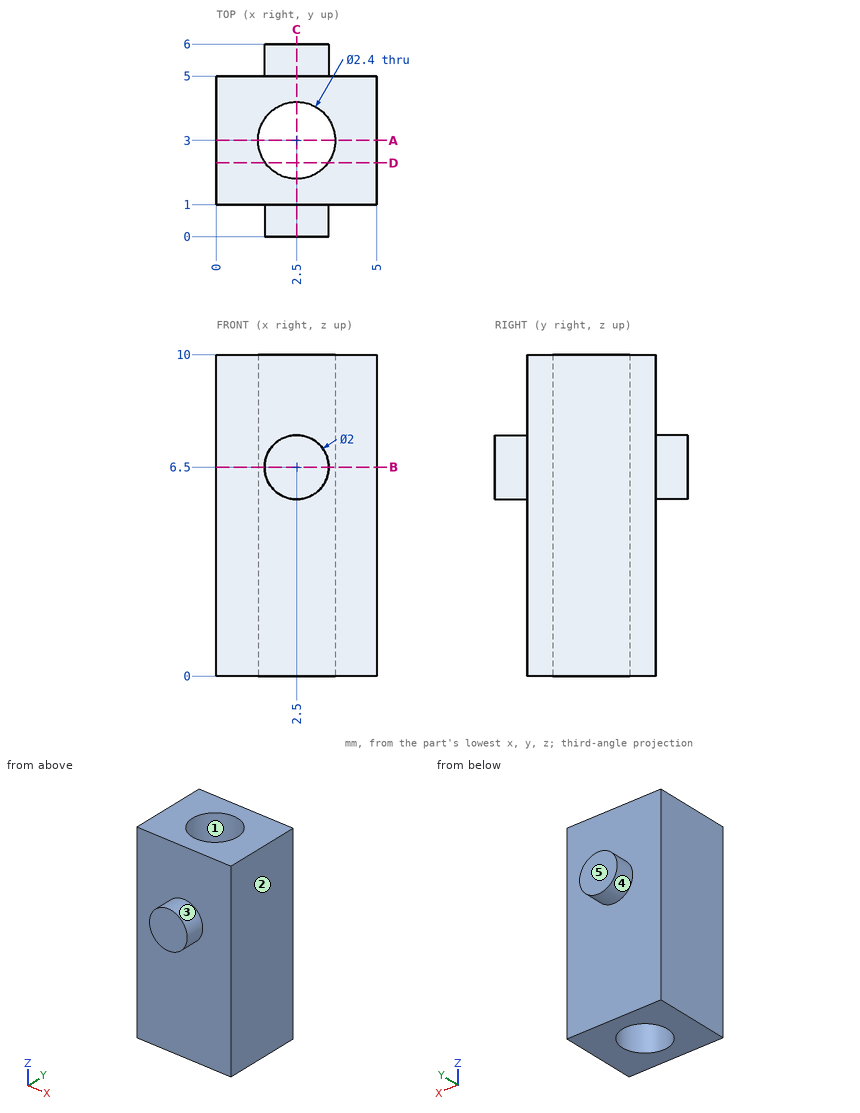
Job drawing, mm, ordinate dimensions from the low corner. One solid piece. A direction names the side the tool comes from. Round coordinates to 2 decimals unless told otherwise and drop trailing zeros. Write each loop counter-clockwise with the first axis right and the second up, starting at its lowest first coordinate (ties: lowest second). Pieces come first, ordered by that corner, then holes. Notation, with made-up numbers: (10, -18) -> (56, -18) arc R22 ccw to (56, 12) -> close; hole circle Ø4 at (13, -6.75). An arc over 180 degrees is marked (long way). Answer as CSV lines item,"result".
1. Mould opens along X. For the marked faces 1, 2 and 3 say: +X half, -X half, draft (parallel to the pull), parting line (faces both ways), or undercut.
Resolved:
face 1,"undercut"
face 2,"+X half"
face 3,"parting line"
2. Drill centre lines: line 1 (X direction, y = 3, z = 5); line 2 (Y direction, x = 2.5, z = 4); line 3 (Y direction, x = 4.65, z = 2). Where is each one in solid material? Low to high.
Resolved:
line 1,"0 to 1.3, 3.7 to 5"
line 2,"1 to 1.8, 4.2 to 5"
line 3,"1 to 5"
3. Slice it at D-D, the plane y = 2.3. List the corners of the cut face in (x, z), plus the area to 3 significant figures.
Resolved:
outline,"(0, 0) -> (1.53, 0) -> (1.53, 10) -> (0, 10) -> close; (3.47, 0) -> (5, 0) -> (5, 10) -> (3.47, 10) -> close"
area,"30.5 mm²"
4. Slice it at B-B, the plane z = 6.5. List the corners of the cut face in (x, y).
Resolved:
outline,"(0, 1) -> (1.5, 1) -> (1.5, 0) -> (3.5, 0) -> (3.5, 1) -> (5, 1) -> (5, 5) -> (3.5, 5) -> (3.5, 6) -> (1.5, 6) -> (1.5, 5) -> (0, 5) -> close; hole circle Ø2.4 at (2.5, 3)"
5. Slice it at C-C, the plane x = 2.5. List the corners of the cut face in (y, z).
Resolved:
outline,"(0, 5.5) -> (1, 5.5) -> (1, 0) -> (1.8, 0) -> (1.8, 10) -> (1, 10) -> (1, 7.5) -> (0, 7.5) -> close; (4.2, 0) -> (5, 0) -> (5, 5.5) -> (6, 5.5) -> (6, 7.5) -> (5, 7.5) -> (5, 10) -> (4.2, 10) -> close"
6. Slice it at A-A, the plane y = 3. List the corners of the cut face in (x, z), plus the area to 3 significant figures.
Resolved:
outline,"(0, 0) -> (1.3, 0) -> (1.3, 10) -> (0, 10) -> close; (3.7, 0) -> (5, 0) -> (5, 10) -> (3.7, 10) -> close"
area,"26.0 mm²"
7. Tool access for the marked faces 4 and 5: list every direction of +Z, -Z, +X, -X, +Y, -Y with a clear straight run to the whole face (end or side of a thin tool).
Resolved:
face 4,"+Y"
face 5,"+Z, -Z, +X, -X, +Y"
